```python
from build123d import *

# Parameters (mm, degrees)
F1_DEPTH = 210
F2_T     = -5
F3_R     = 7.5548203201
F4_DEPTH = 1


with BuildPart() as f1:
    # F0 (on Top) → F1 (new body)
    with BuildSketch(Plane.XY):
        Polygon((55.9746139076, -72.3302552581), (90.7252430464, -11.5651849096), (72.3302552581, 55.9746139076), (11.5651849096, 90.7252430464), (-55.9746139076, 72.3302552581), (-90.7252430464, 11.5651849096), (-72.3302552581, -55.9746139076), (-11.5651849096, -90.7252430464), align=None)
    extrude(amount=F1_DEPTH)

    # F2
    f2_openings = [f1.faces().sort_by_distance(p)[0] for p in [
        (0, 0, 210),
    ]]
    offset(amount=F2_T, openings=f2_openings)

    # F3 (on face) → F4 (cut)
    with BuildSketch(Plane(origin=(81.5277491522, 22.204714499, 0), x_dir=(-0.2627855398, 0.9648542688, 0), z_dir=(0.9648542688, 0.2627855398, 0))):
        with Locations((0, 111.0091432929)):
            Circle(F3_R)
    extrude(amount=-F4_DEPTH, mode=Mode.SUBTRACT)


solid = f1.part
```
Design review of the part built by this model. Coordinates are the model's own, in mm. A direction names the side the tool comes from. Round coordinates to 2 decimals unless told otherwise and drop trailing zeros. Write each loop counter-clockwise with the first axis right and the second up, starting at its lowest first coordinate (ties: lowest second). Pieces come first, ordered by that corner, then holes. Notation, with made-up numbers: (62, 43.5) -> (120, 43.5) arc R4 ccw to (120, 47.5) -> close; hole circle Ø9 at (80, 86.5). An arc over 180 degrees is marked (long way). Answer in a Markdown table with one row per item.
Q1. For faces 1 (the face through (-81.657, -21.732, 103.53)), 2 (the face through (-20.446, 76.825, 106.065)), list the 3-axis set-ups (+Z, -Z, +X, -X, +Y, -Y) from which the entire face can be reached by the end or side of a thin tool; tool diameter is ignored.
The answers:
| item | result |
|---|---|
| face 1 | +Z, -Z, -X, -Y |
| face 2 | +Z |
Q2. Draft analysis for pull direction Z (two halves, no side actions). For faces 3 (the face through (80.6, 21.8, 111.1)), 4 (the face through (-68.78, 39.87, 106.06)), 5 (the face through (-1, 1, 0)), state which applies: +Z half, -Z half, draft (parallel to the pull), parting line (faces both ways), or undercut.
The answers:
| item | result |
|---|---|
| face 3 | undercut |
| face 4 | draft |
| face 5 | -Z half |
Q3. Take a section at A-A, the plane z = 30.5. State the section outline as (x, y) points.
The answers:
| item | result |
|---|---|
| outline | (-90.73, 11.57) -> (-72.33, -55.97) -> (-11.57, -90.73) -> (55.97, -72.33) -> (90.73, -11.57) -> (72.33, 55.97) -> (11.57, 90.73) -> (-55.97, 72.33) -> close; hole (-85.36, 10.88) -> (-68.05, -52.66) -> (-10.88, -85.36) -> (52.66, -68.05) -> (85.36, -10.88) -> (68.05, 52.66) -> (10.88, 85.36) -> (-52.66, 68.05) -> close |
Q4. To check wall thickness, follow L1, parallel to Z at x = 31.5, y = 43; L2, parallel to X at y = -22, z = 68.5; L3, parallel to X at y = 13.5, z = 98.5. State the ranges of each line that lie inside material, in increasing order. Write a range as [from, to].
The answers:
| item | result |
|---|---|
| L1 | [0, 5] |
| L2 | [-81.58, -76.4], [79, 84.76] |
| L3 | [-89.62, -83.86], [78.72, 83.9] |
Q5. Clearance check with flat-ended pins moving along their axes: pin 1 Ø3 at (x, z) = (-60, 50) entering from +Y; pin 2 Ø8 at (x, z) = (39, 162) entering from -Y; pin 3 Ø8 at (y, z) = (-5.5, 76) entering from -X; pin 4 Ø5 at (x, y) = (-11, -64.5) entering from -Z. State where each tip first meets the part, or that it passes through.
The answers:
| item | result |
|---|---|
| pin 1 | y = 67.91 |
| pin 2 | y = -78.04 |
| pin 3 | x = -87.17 |
| pin 4 | z = 0 |
Q6. Take a section at B-B, the plane y = -20.5. State the section outline as (x, z) points, then the cut area to 3 significant figures.
The answers:
| item | result |
|---|---|
| outline | (-81.99, 0) -> (85.62, 0) -> (85.62, 210) -> (79.86, 210) -> (79.86, 5) -> (-76.81, 5) -> (-76.81, 210) -> (-81.99, 210) -> close |
| area | 3,080 mm² |
Q7. Take a section at C-C, the plane x = -40.5. State the section outline as (y, z) points, then the cut area to 3 significant figures.
The answers:
| item | result |
|---|---|
| outline | (-74.18, 0) -> (76.54, 0) -> (76.54, 210) -> (71.36, 210) -> (71.36, 5) -> (-68.42, 5) -> (-68.42, 210) -> (-74.18, 210) -> close |
| area | 3,000 mm² |
